Part model, mm, in its own coordinate system. Face numbers are marked on the shaded views. Coordinates: 2 decimals unless noted, no trailing zeros. Write each loop counter-clockwise with the first axis right and the second up, starting at its lowest first coordinate (ties: lowest second). Pieces come first, ordered by that corner, then holes. Notation, with made-up numbers: (51, -17.5) -> (92, -17.5) arc R29 cw to (92, 8.5) -> close; hole circle Ø1 at (-12.5, -12.75). An arc over 180 degrees is marked (long way). Write item = value, one per line. Start each with the question number.
Q1. Pull direction Z, two halves, no side cores. Call the marked faces 1 and 2: released by +Z, released by -Z, zero draft, split by the parting line, or undercut.
Q2. Band-saw the part on C-C, the plane x = -16. List the corners of the cut face in (y, z).
Q3. Probe line 1 (Y direction, x = -17, z = 2.5); line 2 (X direction, y = 13.5, z = -19.5); line 3 (Y direction, x = 7, z = -1). List the from-to ranges inside material, lowest first.
Q4. Pin check, flat tips, straight feed: P1, Ø10, axis at x = 10.5, y = 18.5, coming from the -Z side; P2, Ø1, axis at x = 20.5, z = 10.5, coming from the +Y side; P3, Ø5, axis at x = -16, y = 19, coming from the +Z side; P4, Ø8, axis at x = -2, z = -20, coming from the +Y side. Stop position of each tip, or through.
Q5. Band-saw the part on D-D, the plane x = -2. List the corners of the cut face in (y, z), plus the area to 3 significant figures.
Q6. Band-saw the part on A-A, the plane z = 0. List the corners of the cut face in (x, y).
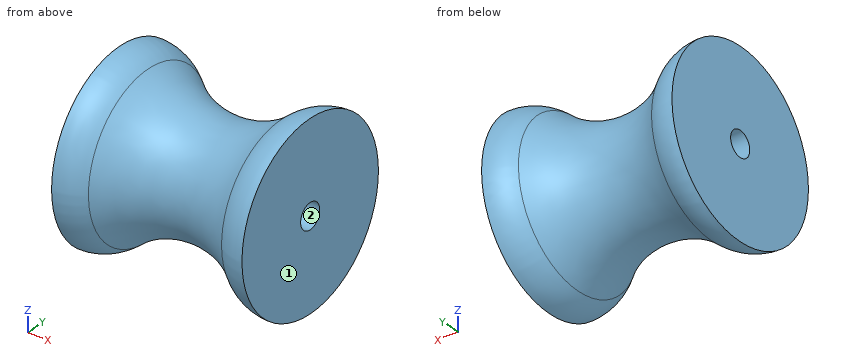
Autodesk Inventor part; units mm, degrees
ref_plane "YZ Plane" through (0, 0, 0) normal (1, 0, 0) x (0, 1, 0)
ref_plane "XZ Plane" through (0, 0, 0) normal (0, 1, 0) x (-1, 0, 0)
ref_plane "XY Plane" through (0, 0, 0) normal (0, 0, 1) x (1, 0, 0)
sketch "Sketch1" plane through (0, 0, 0) normal (0, 1, 0) x (-1, 0, 0)
  line L0 (21.35, -25) -> (26.35, -25)
  line L1 (-21.35, -25) -> (-26.35, -25)
  arc A0 (21.35, -25) -> (-21.35, -25) centre (0, -42.7911) ccw
  line L2 (26.35, 0) -> (-26.35, 0)
  line L3 (-26.35, 0) -> (-26.35, -25)
  line L4 (26.35, 0) -> (26.35, -25)
  point P0 (0, 0)
  dimension "d2" = 5
  dimension "d4" = 5
revolve "Revolution1" add sketch "Sketch1" angle 360 about axis through (-26.35, 0, 0) along (1, 0, 0)
sketch "Sketch2" plane through (-26.35, 0, 0) normal (-1, 0, 0) x (0, 0, 1)
  circle A0 centre (0, 0) radius 25
  circle A1 centre (0, 0) radius 3.5
  dimension "d8" = 7
extrude "Extrusion1" cut sketch "Sketch2" against normal blind 52.7 contours A1
fillet "Fillet2" radius 12 2 edges at (-21.35, 0, 25) (21.35, 0, 25)
properties part number "vystuha_hridel_nahore"
Ans:
q1.face_1 = zero draft
q1.face_2 = undercut
q2.outline = circle Ø40.14 at (0, 0); hole circle Ø7 at (0, 0)
q3.line_1 = -20.66 to -2.45, 2.45 to 20.66
q3.line_2 = -26.35 to -20.98, 20.98 to 26.35
q3.line_3 = -15.86 to -3.35, 3.35 to 15.86
q4.P1 = -11.49
q4.P2 = 21.37
q4.P3 = 12.73
q4.P4 = through
q5.outline = circle Ø30.14 at (0, 0); hole circle Ø7 at (0, 0)
q5.area = 675 mm2
q6.outline = (-26.35, -25) arc R12 ccw to (-18.42, -21.98) arc R27.79 cw to (18.42, -21.98) arc R12 ccw to (26.35, -25) -> (26.35, -3.5) -> (-26.35, -3.5) -> close; (-26.35, 3.5) -> (26.35, 3.5) -> (26.35, 25) arc R12 ccw to (18.42, 21.98) arc R27.79 cw to (-18.42, 21.98) arc R12 ccw to (-26.35, 25) -> close
